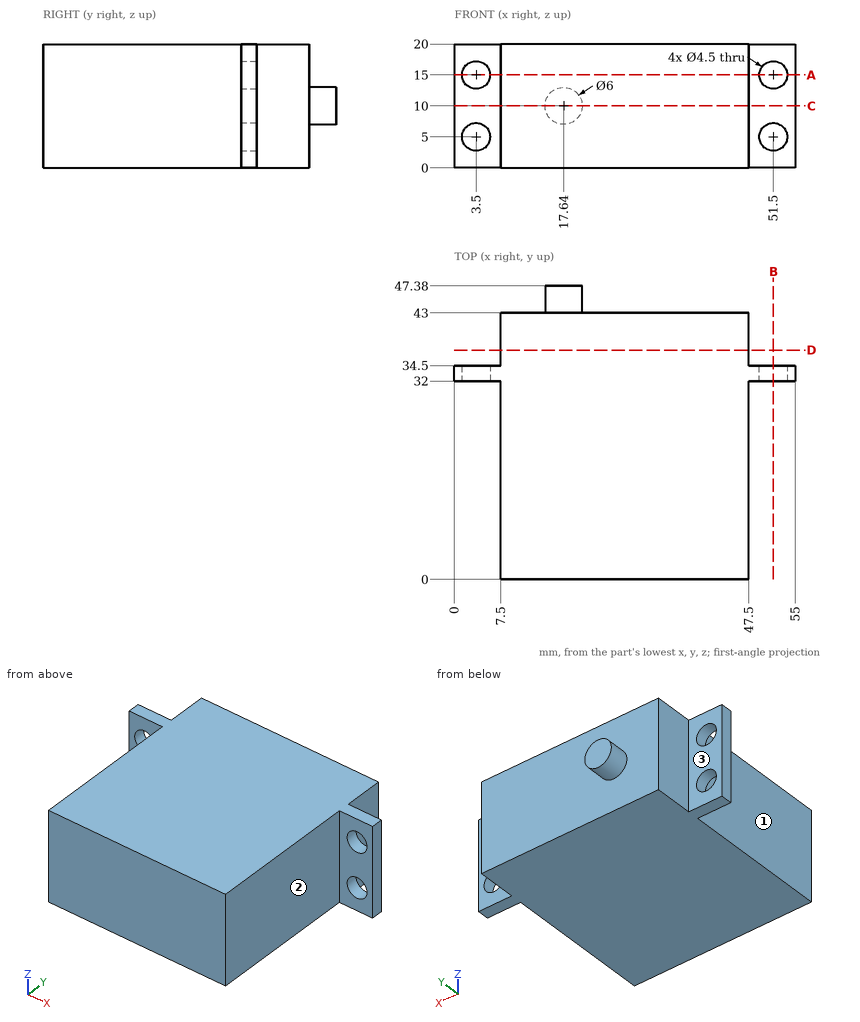
Geometry check sheet. Reference: drawing and pictorial views, mm from the part's lowest x, y, z. A direction names the side the tool comes from. Coordinates: 2 decimals unless noted, no trailing zeros. Order: outer loops, then holes, each group sorted by start corner. A loop starts at its lowest first (then second) coordinate and runs counter-clockwise, first axis right, second up. Notation, with made-up numbers: (75, -21.75) - (96, -21.75) arc R14 cw to (96, 5.25) - close; hole circle Ø8 at (-8.75, 58). An arc over 180 degrees is marked (long way). Answer in a Markdown table with one row per item. Add a question column.
1) Set-up check for the marked faces 1, 2 and 3: record each of +Z, -Z, +X, -X, +Y, -Y from which the full face is reachable in a straight line by a thin tool's end or side.
2) Cross-section at A-A, the plane z = 15. Record the cut outline in (x, y).
3) Material ranges on line 1 along Z through (x, y) = (51.5, 33.9); line 2 along X through (y, z) = (32.65, 15); line 3 along X through (y, z) = (26, 6.75), recorded low to high. Write a range as [from, to].
4) Gauge pin test, flat ends, axial feed: P1, Ø9.5, axis at y = 40, z = 10, coming from the -X side; P2, Ø10, axis at x = 33, z = 7, coming from the +Y side; P3, Ø2, axis at x = 4, z = 7.5, coming from the +Y side. Record the tip position at first contact, or that the pin passes through.
5) Cross-section at B-B, the plane x = 51.5. Record the cut outline in (y, z), then the cut area to 3 significant figures.
6) Cross-section at D-D, the plane y = 37. Record the cut outline in (x, z), then the cut area to 3 significant figures.
7) Cross-section at C-C, the plane z = 10. Record the cut outline in (x, y), then the cut area to 3 significant figures.
Check result:
| question | item | result |
|---|---|---|
| 1 | face 1 | +Z, -Z, -X, -Y |
| 1 | face 2 | +Z, -Z, +X, -Y |
| 1 | face 3 | +Z, -Z, -X, +Y |
| 2 | outline | (0, 32) - (1.25, 32) - (1.25, 34.5) - (0, 34.5) - close; (5.75, 32) - (7.5, 32) - (7.5, 0) - (47.5, 0) - (47.5, 32) - (49.25, 32) - (49.25, 34.5) - (47.5, 34.5) - (47.5, 43) - (7.5, 43) - (7.5, 34.5) - (5.75, 34.5) - close; (53.75, 32) - (55, 32) - (55, 34.5) - (53.75, 34.5) - close |
| 3 | line 1 | z = [0, 2.75], [7.25, 12.75], [17.25, 20] |
| 3 | line 2 | x = [0, 1.25], [5.75, 49.25], [53.75, 55] |
| 3 | line 3 | x = [7.5, 47.5] |
| 4 | P1 | stops at x = 7.5 |
| 4 | P2 | stops at y = 43 |
| 4 | P3 | stops at y = 34.5 |
| 5 | outline | (32, 0) - (34.5, 0) - (34.5, 2.75) - (32, 2.75) - close; (32, 7.25) - (34.5, 7.25) - (34.5, 12.75) - (32, 12.75) - close; (32, 17.25) - (34.5, 17.25) - (34.5, 20) - (32, 20) - close |
| 5 | area | 27.5 mm² |
| 6 | outline | (7.5, 0) - (47.5, 0) - (47.5, 20) - (7.5, 20) - close |
| 6 | area | 800 mm² |
| 7 | outline | (0, 32) - (7.5, 32) - (7.5, 0) - (47.5, 0) - (47.5, 32) - (55, 32) - (55, 34.5) - (47.5, 34.5) - (47.5, 43) - (20.64, 43) - (20.64, 47.38) - (14.64, 47.38) - (14.64, 43) - (7.5, 43) - (7.5, 34.5) - (0, 34.5) - close |
| 7 | area | 1,780 mm² |
